Check sheet for the drawn part. Datum: minimum x, y, z corner. Units: mm. A direction names the side the tool comes from. Coordinates: 2 decimals unless noted, no trailing zeros. Loops run counter-clockwise (first coordinate to the right, second up) from the corner with the lowest first, then second, coordinate; pieces in that order, holes last.
Q1. Sectioned sample at A-A (y = 2.3). Enter the section's corners in (x, z), then the cut area to 3 significant figures.
Q2. Sectioned sample at D-D (z = 18.5). Enter the section's corners in (x, y), then the cut area to 3 significant figures.
Q3. Access from +Z, -Z, +X, -X, +Y, -Y to the whole of each face (thin tool, end or side, straight path). Record for the marked faces 1, 2 and 3.
Q4. Go/stop test with flat-tipped pins: P1, Ø1.5, axis at x = 4.5, y = 0.5, coming from the +Z side; P2, Ø1, axis at y = 2.5, z = 18.5, coming from the -X side; P3, Ø1.6, axis at x = 4.5, z = 20, coming from the -Y side. Record where each tip stops, or that it passes through.
Q5. Sectioned sample at B-B (z = 7). Enter the section's corners in (x, y), then the cut area to 3 significant figures.
Q6. Sectioned sample at C-C (x = 3.5). Enter the section's corners in (y, z), then the cut area to 3 significant figures.
Q7. Material ranges on probe 1 along X at (y, z) = (2.5, 20.5); probe 2 along Z at (x, y) = (2.5, 2.5); probe 3 along Y at (x, z) = (5.5, 17.5), recorded low to high.
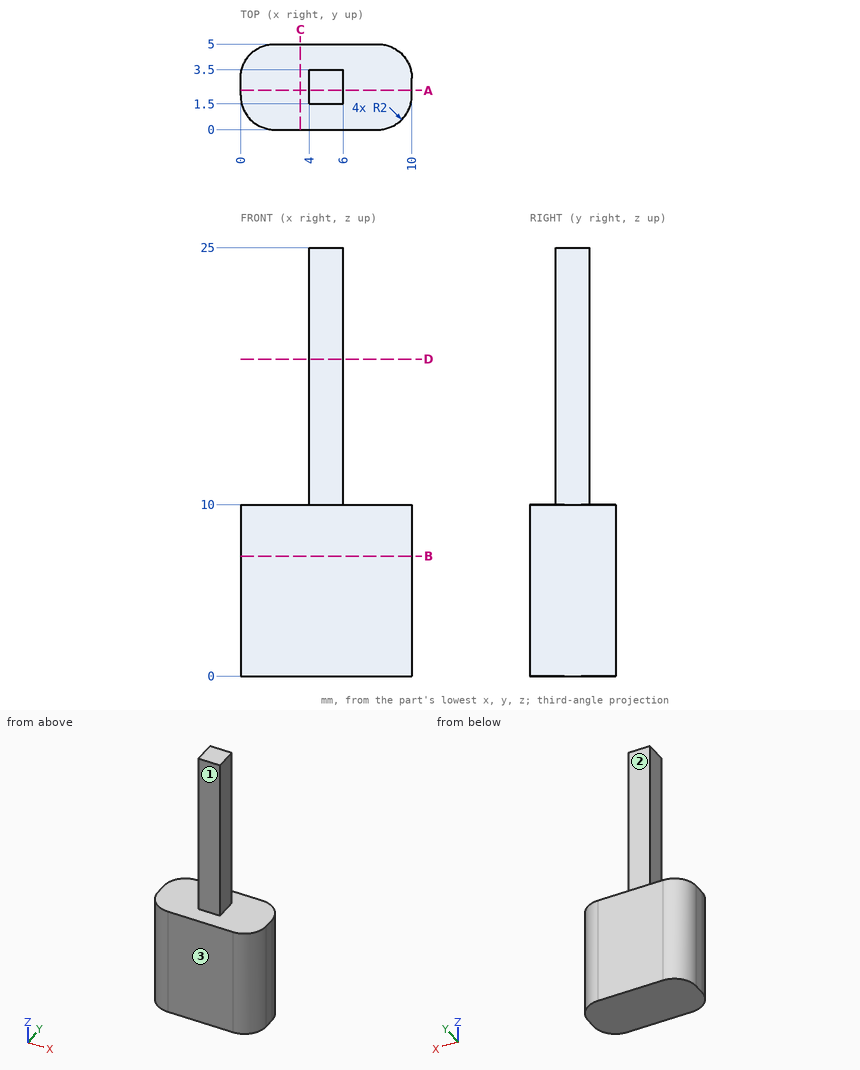
Geometry check:
1. outline: (0, 0) - (10, 0) - (10, 10) - (6, 10) - (6, 25) - (4, 25) - (4, 10) - (0, 10) - close
1. area: 130 mm2
2. outline: (4, 1.5) - (6, 1.5) - (6, 3.5) - (4, 3.5) - close
2. area: 4.00 mm2
3. face 1: +Z, +X, -X, -Y
3. face 2: +Z, +X, -X, +Y
3. face 3: +Z, -Z, +X, -X, -Y
4. P1: stops at z = 10
4. P2: stops at x = 4
4. P3: stops at y = 1.5
5. outline: (0, 2) arc R2 ccw to (2, 0) - (8, 0) arc R2 ccw to (10, 2) - (10, 3) arc R2 ccw to (8, 5) - (2, 5) arc R2 ccw to (0, 3) - close
5. area: 46.6 mm2
6. outline: (0, 0) - (5, 0) - (5, 10) - (0, 10) - close
6. area: 50.0 mm2
7. probe 1: x = 4 to 6
7. probe 2: z = 0 to 10
7. probe 3: y = 1.5 to 3.5
